Source: CAD feature listing. Evaluate the final solid. Frame: model axes, mm. Round coordinates to 2 decimals unless told otherwise and drop trailing zeros. Loops run counter-clockwise (first coordinate to the right, second up) from the corner with the lowest first, then second, coordinate; pieces in that order, holes last.
(1) Section D-D, the plane z = -54. Return the cut outline in (x, y), plus the area to 3 significant figures.
(2) First-contact query: pin 1 Ø7 at (x, z) = (-39.607, -50.472) entering from +Y; pin 2 Ø0.8 at (y, z) = (0.5, -28.5) entering from +X; pin 3 Ø0.5 at (x, y) = (-7, 1) entering from -Z. Flat tips, straight axial feed; report the tip coordinate or a pass-through.
(3) Material intervals for probe 1 along X at (y, z) = (0.7, -0.5); probe 2 along Z at (x, y) = (0, 0.9); probe 3 along X at (y, z) = (0.4, -51), sorted ascending.
(4) Section B-B, the plane x = -8. Return the cut outline in (y, z).
(5) Section C-C, the plane y = 0.7. Count the separate pieces of the cut face and the enclosed holes in it, plus the area to 3 significant figures.
(6) Section A-A, the plane z = -76.2. Return the cut outline in (x, y), plus the area to 3 significant figures.
Autodesk Inventor part; units mm, degrees
ref_plane "YZ Plane" through (0, 0, 0) normal (1, 0, 0) x (0, 1, 0)
ref_plane "XZ Plane" through (0, 0, 0) normal (0, 1, 0) x (-1, 0, 0)
ref_plane "XY Plane" through (0, 0, 0) normal (0, 0, 1) x (1, 0, 0)
sketch "main" plane through (0, 0, 0) normal (0, 0, 1) x (1, 0, 0)
  line L0 (12.0188, -14.2552) -> (34.1049, 26.0684)
  circle A0 centre (21.9619, 13.8124) radius 2.1844
  circle A1 centre (31.5972, 36.5815) radius 2.1844
  circle A2 centre (36.4896, 64.2776) radius 2.1844
  line L1 (36.4904, 70.6276) -> (-17.6528, 70.6344)
  circle A3 centre (7.7473, 64.2844) radius 2.1844
  line L2 (7.7507, 48.4162) -> (7.7558, 29.3619)
  arc A4 (7.7507, 48.4162) -> (-1.7768, 57.9386) centre (-1.7743, 48.4136) ccw
  arc A5 (-1.7692, 19.8344) -> (7.7558, 29.3619) centre (-1.7692, 29.3594) ccw
  line L3 (-17.645, 57.9344) -> (-1.7768, 57.9386)
  arc A6 (-17.6528, 70.6344) -> (-17.645, 57.9344) centre (-17.645, 64.2844) ccw
  arc A7 (-17.6527, 19.8344) -> (-21.9541, 8.8131) centre (-17.6527, 13.4844) ccw
  circle A8 centre (7.7473, 13.4844) radius 2.1844
  line L4 (-1.7692, 19.8344) -> (-17.6527, 19.8344)
  arc A9 (4.4483, -15.4983) -> (12.0188, -14.2552) centre (7.7473, -11.9156) ccw
  line L5 (4.4483, -15.4983) -> (-21.9541, 8.8131)
  circle A10 centre (7.7473, -11.9156) radius 2.1844
  circle A11 centre (-17.645, 64.2844) radius 2.1844
  circle A12 centre (-17.6527, 13.4844) radius 2.1844
  arc A13 (40.98, 68.7674) -> (36.4904, 70.6276) centre (36.4896, 64.2776) ccw
  line L6 (40.98, 68.7674) -> (47.2524, 62.495)
  line L7 (40.98, 68.7674) -> (49.8505, 68.7674) construction
  line L8 (47.9374, 59.0271) -> (34.6865, 27.2778)
  arc A14 (34.1049, 26.0684) -> (34.6865, 27.2778) centre (22.9663, 32.1693) ccw
  arc A15 (47.9374, 59.0271) -> (47.2524, 62.495) centre (45.0073, 60.25) ccw
  point P0 (10.5119, 26.5593)
  point P1 (34.4277, 26.6577)
  dimension "d1" = 9.7405
  dimension "d2" = 4.3688
  dimension "d3" = 4.3688
  dimension "d4" = 4.3688
  dimension "d5" = 4.3688
  dimension "d6" = 4.3688
  dimension "d10" = 50.8
  dimension "d11" = 50.8
  dimension "d13" = 6.35
  dimension "d20" = 45
  dimension "d21" = 12.7
  dimension "d22" = 3.175
sketch "Sketch1" plane through (0, 0, 0) normal (0, 1, 0) x (-1, 0, 0)
  line L0 (29.6638, -78.5396) -> (51.75, -38.2159)
  circle A0 centre (39.607, -50.472) radius 2.1844
  circle A1 centre (49.2422, -27.7029) radius 2.1844
  circle A2 centre (54.1346, -0.0068) radius 2.1844
  line L1 (54.1354, 6.3432) -> (-0.0077, 6.35)
  circle A3 centre (25.3923, 0) radius 2.1844
  line L2 (25.3957, -15.8682) -> (25.4009, -34.9224)
  arc A4 (25.3957, -15.8682) -> (15.8682, -6.3457) centre (15.8707, -15.8707) ccw
  arc A5 (15.8759, -44.45) -> (25.4009, -34.9224) centre (15.8759, -34.925) ccw
  line L3 (0, -6.35) -> (15.8682, -6.3457)
  arc A6 (-0.0077, 6.35) -> (0, -6.35) centre (0, 0) ccw
  arc A7 (-0.0077, -44.45) -> (-4.309, -55.4713) centre (-0.0077, -50.8) ccw
  circle A8 centre (25.3923, -50.8) radius 2.1844
  line L4 (15.8759, -44.45) -> (-0.0077, -44.45)
  arc A9 (22.0933, -79.7827) -> (29.6638, -78.5396) centre (25.3923, -76.2) ccw
  line L5 (22.0933, -79.7827) -> (-4.309, -55.4713)
  circle A10 centre (25.3923, -76.2) radius 2.1844
  circle A11 centre (0, 0) radius 2.1844
  circle A12 centre (-0.0077, -50.8) radius 2.1844
  arc A13 (58.625, 4.483) -> (54.1354, 6.3432) centre (54.1346, -0.0068) ccw
  line L6 (58.625, 4.483) -> (64.8974, -1.7894)
  line L7 (58.625, 4.483) -> (67.4955, 4.483) construction
  line L8 (65.5824, -5.2573) -> (52.3315, -37.0066)
  arc A14 (51.75, -38.2159) -> (52.3315, -37.0066) centre (40.6113, -32.1151) ccw
  arc A15 (65.5824, -5.2573) -> (64.8974, -1.7894) centre (62.6524, -4.0344) ccw
extrude "Extrusion1" add sketch "Sketch1" along normal blind 1.5875
properties part number "Funnel Gusset Back Improved V2" material "Acetal Resin, White"
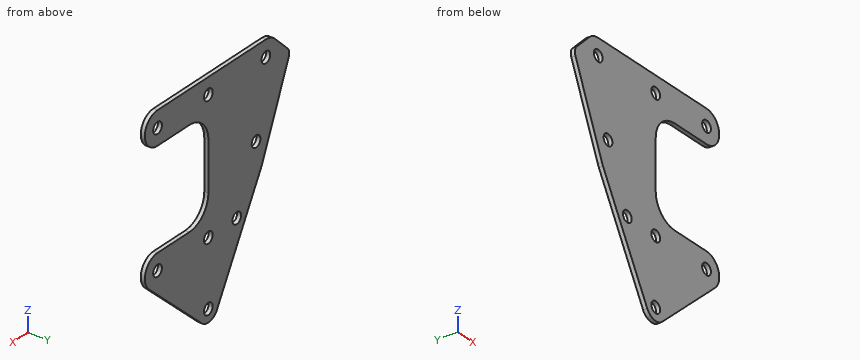
Output values:
1. outline: (-43.1, 0) - (5.49, 0) - (5.49, 1.59) - (-43.1, 1.59) - close
1. area: 77.1 mm2
2. pin 1: stops at y = 1.59
2. pin 2: stops at x = -25.4
2. pin 3: stops at z = -66.11
3. probe 1: x = -63.61 to -56.26, -52.01 to -27.52, -23.27 to -2.13, 2.13 to 6.33
3. probe 2: z = -59.44 to -52.98, -48.62 to -44.45, -6.35 to -2.18, 2.18 to 6.35
3. probe 3: x = -44.75 to -41.73, -37.49 to -27.57, -23.22 to -2.17, 2.18 to 6.35
4. outline: (0, -66.81) - (1.59, -66.81) - (1.59, -44.45) - (0, -44.45) - close; (0, -6.35) - (1.59, -6.35) - (1.59, 6.35) - (0, 6.35) - close
5. separate pieces: 1
5. enclosed holes: 8
5. area: 3,200 mm2
6. outline: (-30.95, 0) - (-27.58, 0) - (-27.58, 1.59) - (-30.95, 1.59) - close; (-23.21, 0) - (-18.2, 0) - (-18.2, 1.59) - (-23.21, 1.59) - close
6. area: 13.3 mm2
